```python
from build123d import *

# Parameters (mm, degrees)
SKETCH2_R           = 2.54
BOSS_EXTRUDE1_DEPTH = 2.54


with BuildPart() as part:
    # Sketch2 → Boss-Extrude1 (new body)
    with BuildSketch(Plane.XY):
        with BuildLine():
            Line((317.5, 62.23), (317.5, 121.92))
            ThreePointArc((317.5, 121.92), (318.987897552, 125.512102448), (322.58, 127))
            Line((322.58, 127), (337.82, 127))
            ThreePointArc((337.82, 127), (341.412102448, 125.512102448), (342.9, 121.92))
            Line((342.9, 121.92), (342.9, 87.63))
            ThreePointArc((342.9, 87.63), (344.387897552, 84.037897552), (347.98, 82.55))
            Line((347.98, 82.55), (426.72, 82.55))
            ThreePointArc((426.72, 82.55), (430.312102448, 84.037897552), (431.8, 87.63))
            Line((431.8, 87.63), (431.8, 134.62))
            ThreePointArc((431.8, 134.62), (433.287897552, 138.212102448), (436.88, 139.7))
            Line((436.88, 139.7), (452.12, 139.7))
            ThreePointArc((452.12, 139.7), (455.712102448, 138.212102448), (457.2, 134.62))
            Line((457.2, 134.62), (457.2, 82.55))
            Line((457.2, 82.55), (457.2, 62.23))
            ThreePointArc((457.2, 62.23), (455.712102448, 58.637897552), (452.12, 57.15))
            Line((452.12, 57.15), (322.58, 57.15))
            ThreePointArc((322.58, 57.15), (318.987897552, 58.637897552), (317.5, 62.23))
        make_face()
        with Locations((444.5, 133.35)):
            Circle(SKETCH2_R, mode=Mode.SUBTRACT)
        with Locations((444.5, 120.65)):
            Circle(SKETCH2_R, mode=Mode.SUBTRACT)
        with Locations((444.5, 107.95)):
            Circle(SKETCH2_R, mode=Mode.SUBTRACT)
        with Locations((444.5, 95.25)):
            Circle(SKETCH2_R, mode=Mode.SUBTRACT)
        with Locations((444.5, 69.85)):
            Circle(SKETCH2_R, mode=Mode.SUBTRACT)
        with Locations((431.8, 69.85)):
            Circle(SKETCH2_R, mode=Mode.SUBTRACT)
        with Locations((419.1, 69.85)):
            Circle(SKETCH2_R, mode=Mode.SUBTRACT)
        with Locations((406.4, 69.85)):
            Circle(SKETCH2_R, mode=Mode.SUBTRACT)
        with Locations((393.7, 69.85)):
            Circle(SKETCH2_R, mode=Mode.SUBTRACT)
        with Locations((381, 69.85)):
            Circle(SKETCH2_R, mode=Mode.SUBTRACT)
        with Locations((368.3, 69.85)):
            Circle(SKETCH2_R, mode=Mode.SUBTRACT)
        with Locations((355.6, 69.85)):
            Circle(SKETCH2_R, mode=Mode.SUBTRACT)
        with Locations((330.2, 69.85)):
            Circle(SKETCH2_R, mode=Mode.SUBTRACT)
        with Locations((330.2, 82.55)):
            Circle(SKETCH2_R, mode=Mode.SUBTRACT)
        with Locations((330.2, 95.25)):
            Circle(SKETCH2_R, mode=Mode.SUBTRACT)
        with Locations((330.2, 107.95)):
            Circle(SKETCH2_R, mode=Mode.SUBTRACT)
        with Locations((330.2, 120.65)):
            Circle(SKETCH2_R, mode=Mode.SUBTRACT)
    extrude(amount=BOSS_EXTRUDE1_DEPTH)


solid = part.part
```
Geometry: final body of the model. Coordinates: model frame, mm. A direction names the side the tool comes from. Give positions to 0.01 mm unless a question says otherwise; leave off trailing zeros. Loops run counter-clockwise (first coordinate to the right, second up) from the corner with the lowest first, then second, coordinate; pieces in that order, holes last. Notation, with made-up numbers: (55.25, -11.5) - (90.25, -11.5) arc R17 cw to (90.25, -4.5) - close; hole circle Ø5 at (37, -35.75). An arc over 180 degrees is marked (long way). Answer as CSV lines item,"result". Start each with the question number.
(1) Section query B-B (y = 107.95). Output: boundary loops of the cut face in (x, z).
(2) Section query A-A (x = 330.2). Output: boundary loops of the cut face in (y, z).
(3) Pin query (flat end, axial travel): P1, Ø8, axis at x = 330.2, y = 120.65, coming from the -Z side. Return the tip coordinate at first contact, or that it passes through.
(4) Section query D-D (z = 2.1). Give the number of separate pieces and of enclosed holes in the cut face, and give its area (3 significant figures).
(5) Section query C-C (x = 419.1). Output: boundary loops of the cut face in (y, z).
(6) Reachability of faces 1 (the face through (370.646, 68.877, 1.252)), 2 (the face through (387, 82.55, 1)) from +Z, -Z, +X, -X, +Y, -Y: full face, straight path, thin tool, end or side. Return the list, or none.
(7) Ray query, line 1 along Y through (x, z) = (330.2, 1.8); line 2 along Y through (x, z) = (444.5, 2.05); line 3 along X through (y, z) = (103, 1.7). Return the intervals inside material, ascending. Write a range as [from, to].
(8) Mould query, pull axis X, two halves, no side actions, for faces 3 (the face through (433.249, 138.172, 1.252)), 4 (the face through (330, 127, 1)), 5 (the face through (417.084, 68.304, 1.252)). Classes: +X half, -X half, draft (parallel to the pull), parting line (faces both ways), or undercut.
Worked answers:
1,outline,"(317.5, 0) - (327.66, 0) - (327.66, 2.54) - (317.5, 2.54) - close; (332.74, 0) - (342.9, 0) - (342.9, 2.54) - (332.74, 2.54) - close; (431.8, 0) - (441.96, 0) - (441.96, 2.54) - (431.8, 2.54) - close; (447.04, 0) - (457.2, 0) - (457.2, 2.54) - (447.04, 2.54) - close"
2,outline,"(57.15, 0) - (67.31, 0) - (67.31, 2.54) - (57.15, 2.54) - close; (72.39, 0) - (80.01, 0) - (80.01, 2.54) - (72.39, 2.54) - close; (85.09, 0) - (92.71, 0) - (92.71, 2.54) - (85.09, 2.54) - close; (97.79, 0) - (105.41, 0) - (105.41, 2.54) - (97.79, 2.54) - close; (110.49, 0) - (118.11, 0) - (118.11, 2.54) - (110.49, 2.54) - close; (123.19, 0) - (127, 0) - (127, 2.54) - (123.19, 2.54) - close"
3,P1,"stops at z = 0"
4,separate pieces,"1"
4,enclosed holes,"17"
4,area,"5,760 mm^2"
5,outline,"(57.15, 0) - (67.31, 0) - (67.31, 2.54) - (57.15, 2.54) - close; (72.39, 0) - (82.55, 0) - (82.55, 2.54) - (72.39, 2.54) - close"
6,face 1,"+Z, -Z"
6,face 2,"+Z, -Z, +Y"
7,line 1,"y = [57.15, 67.31], [72.39, 80.01], [85.09, 92.71], [97.79, 105.41], [110.49, 118.11], [123.19, 127]"
7,line 2,"y = [57.15, 67.31], [72.39, 92.71], [97.79, 105.41], [110.49, 118.11], [123.19, 130.81], [135.89, 139.7]"
7,line 3,"x = [317.5, 342.9], [431.8, 457.2]"
8,face 3,"-X half"
8,face 4,"draft"
8,face 5,"undercut"
